Here's how the part is built. I have some questions about the finished solid (model axes, mm). Face numbers are marked on the shaded views. A direction names the side the tool comes from. Round coordinates to 2 decimals unless told otherwise and drop trailing zeros. Loops run counter-clockwise (first coordinate to the right, second up) from the corner with the lowest first, then second, coordinate; pieces in that order, holes last. Notation, with made-up numbers: (17, -27.75) -> (27, -27.75) arc R28 ccw to (27, -3.75) -> close; hole circle Ø7 at (80, -7). An arc over 180 degrees is marked (long way). Use CSV: the item, a comma, the result in double quotes. Start each with the question number.
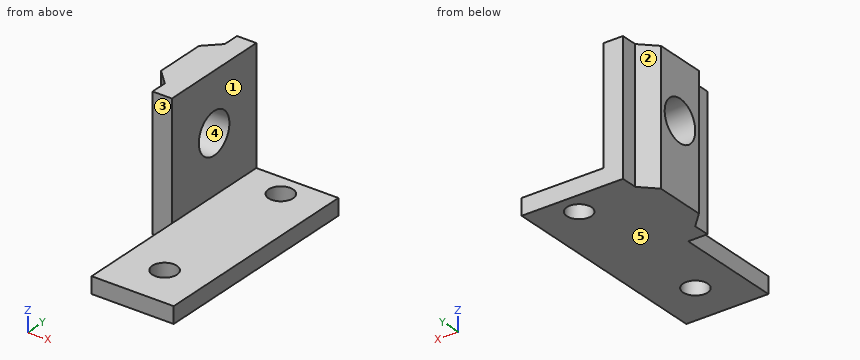
from build123d import *

# Parameters (mm, degrees)
SKETCH1_W           = 10
SKETCH1_H           = 26.92
SKETCH1_R           = 1.5
BOSS_EXTRUDE1_DEPTH = 2
BOSS_EXTRUDE2_DEPTH = 16
SKETCH5_R           = 2.5
CUT_EXTRUDE1_DEPTH  = 16


with BuildPart() as part:
    # Sketch1 → Boss-Extrude1 (new body)
    with BuildSketch(Plane.XY):
        with Locations((5, 13.46)):
            Rectangle(SKETCH1_W, SKETCH1_H)
        with Locations((5, 24.22)):
            Circle(SKETCH1_R, mode=Mode.SUBTRACT)
        with Locations((5, 5.22)):
            Circle(SKETCH1_R, mode=Mode.SUBTRACT)
    extrude(amount=BOSS_EXTRUDE1_DEPTH)

    # Sketch2 → Boss-Extrude2 (add)
    with BuildSketch(Plane(origin=(0, 0, 0), x_dir=(-1, 0, 0), z_dir=(0, 0, -1))):
        Polygon((2.35, 24.92), (4.15, 23.12), (4.15, 16.92), (2.35, 15.12), (2.35, 13.12), (0, 13.12), (0, 15.12), (0, 24.92), (0, 26.92), (2.35, 26.92), align=None)
    extrude(amount=-BOSS_EXTRUDE2_DEPTH)

    # Sketch5 → Cut-Extrude1 (cut)
    with BuildSketch(Plane(origin=(0, 0, 0), x_dir=(0, 0, -1), z_dir=(1, 0, 0))):
        with Locations(Location((-9, 20.02, 0), (0, 0, 90))):
            Circle(SKETCH5_R)
    extrude(amount=-CUT_EXTRUDE1_DEPTH, mode=Mode.SUBTRACT)


solid = part.part
Q1. For the marked faces 1 and 2, which set-ups out of +Z, -Z, +X, -X, +Y, -Y let a thin tool reach every point of the face, with its end or its side?
Q2. I want a section at B-B, the plane y = 5.22. List the corners of the cut face in (x, z) for me.
Q3. If we mould it in two halves opening along Z, with no side actions, what happens to the marked faces 3, 4 and 5? For each: pulls with the +Z half, pulls with the -Z half, needs draft (parallel to the pull), parting line crosses it, or undercut.
Q4. I want a section at C-C, the plane x = 5. List the corners of the cut face in (y, z) for me.
Q5. Will these pins go through, and if not, where does the flat tip stop? pin 1 Ø1.2 at (x, z) = (-1, 9) entering from -Y; pin 2 Ø5 at (x, y) = (4.5, 17) entering from +Z; pin 3 Ø0.6 at (y, z) = (9.5, 1) entering from -X.
Q6. I want a section at D-D, the plane z = 2.5. List the corners of the cut face in (x, y) for me.
Q7. I want a section at A-A, the plane z = 9. List the corners of the cut face in (x, y) for me, then the cut area to 3 significant figures.
Q8. I need wall thicknesses on line 1 along Y through (x, z) = (5, 0.8); line 2 along Z through (x, y) = (-3.3, 20.02); line 3 along Z through (x, y) = (3.75, 19). Which ranges of each line are inside material? Lowest first, please.
Values found:
1,face 1,"+Z, +X, +Y, -Y"
1,face 2,"+Z, -Z, -X, +Y"
2,outline,"(0, 0) -> (3.5, 0) -> (3.5, 2) -> (0, 2) -> close; (6.5, 0) -> (10, 0) -> (10, 2) -> (6.5, 2) -> close"
3,face 3,"needs draft"
3,face 4,"undercut"
3,face 5,"pulls with the -Z half"
4,outline,"(0, 0) -> (3.72, 0) -> (3.72, 2) -> (0, 2) -> close; (6.72, 0) -> (22.72, 0) -> (22.72, 2) -> (6.72, 2) -> close; (25.72, 0) -> (26.92, 0) -> (26.92, 2) -> (25.72, 2) -> close"
5,pin 1,"y = 13.12"
5,pin 2,"z = 2"
5,pin 3,"x = 0"
6,outline,"(-4.15, 16.92) -> (-2.35, 15.12) -> (-2.35, 13.12) -> (0, 13.12) -> (0, 26.92) -> (-2.35, 26.92) -> (-2.35, 24.92) -> (-4.15, 23.12) -> close"
7,outline,"(-4.15, 16.92) -> (-2.35, 15.12) -> (-2.35, 13.12) -> (0, 13.12) -> (0, 17.52) -> (-4.15, 17.52) -> close; (-4.15, 22.52) -> (0, 22.52) -> (0, 26.92) -> (-2.35, 26.92) -> (-2.35, 24.92) -> (-4.15, 23.12) -> close"
7,area,"26.1 mm2"
8,line 1,"0 to 3.72, 6.72 to 22.72, 25.72 to 26.92"
8,line 2,"0 to 6.5, 11.5 to 16"
8,line 3,"0 to 2"
